Answer from the drawing. Dimensions are ordinates in mm from the lowest x, y and z of the part. A direction names the side the tool comes from. Give positions to 0.01 mm unless a question says otherwise; leave off trailing zeros. Order: outer loops, then holes, each group sorted by start corner. A loop starts at its lowest first (then second) coordinate and runs counter-clockwise, first axis right, second up.
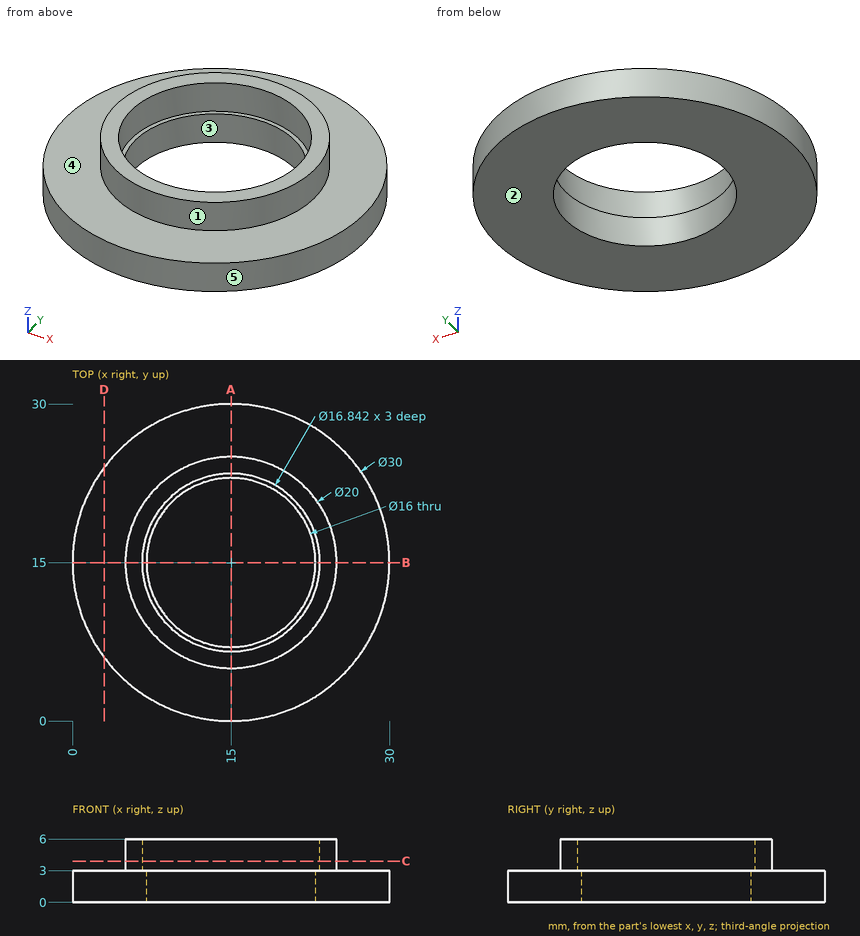
1. Given P1, Ø1.5, axis at x = 8, z = 2.5, coming from the +Y side; P2, Ø2, axis at y = 20, z = 2, coming from the -X side; P3, Ø1.5, axis at x = 27, y = 25.5, coming from the -Z side, each flat-ended and moving along its own axis, determine where each tip first touches the part or whether it passes through.
Findings below:
P1: stops at y = 28.64
P2: stops at x = 0.54
P3: passes through
2. The part is cut by section D-D (x = 3). Write down the section's boundary in (y, z), then the cut area to 3 significant figures.
Findings below:
outline: (6, 0) - (24, 0) - (24, 3) - (6, 3) - close
area: 54.0 mm2
3. The part is cut by section A-A (x = 15). Write down the section's boundary in (y, z).
Findings below:
outline: (0, 0) - (7, 0) - (7, 3) - (6.58, 3) - (6.58, 6) - (5, 6) - (5, 3) - (0, 3) - close; (23, 0) - (30, 0) - (30, 3) - (25, 3) - (25, 6) - (23.42, 6) - (23.42, 3) - (23, 3) - close
4. Which of the six approach directions +Z, -Z, +X, -X, +Y, -Y give full straight-line access (tool end or side, diameter ignored) to the marked faces 1 and 2?
Findings below:
face 1: +Z
face 2: -Z, +X, -X, +Y, -Y
5. Straight lines are drawn through the part: probe 1 along Y at (x, z) = (15, 1.3); probe 2 along Y at (x, z) = (15, 4.2); probe 3 along Z at (x, y) = (20, 5.25). For each, find the intervals that lie inside material, in ascending order.
Findings below:
probe 1: y = 0 to 7, 23 to 30
probe 2: y = 5 to 6.58, 23.42 to 25
probe 3: z = 0 to 3
6. The part is cut by section C-C (z = 3.9). Write down the section's boundary in (x, y).
Findings below:
outline: circle Ø20 at (15, 15); hole circle Ø16.84 at (15, 15)
7. The mould has two halves that part along Y. Classify the marked faces 3, 4 and 5: pulls with the +Y half, pulls with the -Y half, needs draft (parallel to the pull), parting line crosses it, or undercut.
Findings below:
face 3: undercut
face 4: needs draft
face 5: parting line crosses it
